```python
from build123d import *

# Parameters (mm, degrees)
ESQUISSE1_W               = 60.5
ESQUISSE1_H               = 64
BOSS_EXTRU_1_DEPTH        = 30
ESQUISSE2_R               = 4.5
ENL_V_MAT_EXTRU_1_DEPTH   = 32
ENL_V_MAT_EXTRU_2_REACH   = 55.283
ESQUISSE4_W               = 51.1
ESQUISSE4_H               = 83.557669167
ESQUISSE5_R               = 10.5
ENL_V_MAT_EXTRU_3_DEPTH   = 2
ESQUISSE6_R               = 10
ENL_V_MAT_EXTRU_4_DEPTH   = 4.7
ESQUISSE7_W               = 47
ESQUISSE7_H               = 57
BOSS_EXTRU_2_DEPTH        = 30
ENL_V_MAT_EXTRU_5_DEPTH   = 30
ENL_V_MAT_EXTRU_6_DEPTH   = 8.25
ESQUISSE11_W              = 5
ESQUISSE11_H              = 40.5
BOSS_EXTRU_3_DEPTH        = 5
ESQUISSE12_R              = 0.5
ENL_V_MAT_EXTRU_7_DEPTH   = 15
TROU_TARAUD_M2X0_42_D     = 1.6
TROU_TARAUD_M2X0_42_DEPTH = 17
TROU_TARAUD_M2X0_42_TIP   = 0.480688495
ENL_V_MAT_EXTRU_8_REACH   = 113.72
ESQUISSE22_W              = 82.97203866
ESQUISSE22_H              = 67.875780224
ENL_V_MAT_EXTRU_10_DEPTH  = 30
ESQUISSE23_W              = 55
ESQUISSE23_H              = 5
ESQUISSE23_H_2            = 4.9
BOSS_EXTRU_4_DEPTH        = 30
ENL_V_START               = -62
ESQUISSE24_R              = 10
ENL_V_MAT_EXTRU_11_DEPTH  = 62
ENL_V_MAT_EXTRU_12_REACH  = 111.597
ESQUISSE26_R              = 10.5
ESQUISSE26_R_2            = 4.5
BOSS_EXTRU_5_DEPTH        = 5
ESQUISSE27_R              = 10.5
ENL_V_MAT_EXTRU_13_DEPTH  = 2.5
ESQUISSE28_W              = 21.53784572
ESQUISSE28_H              = 33.22443827
ENL_V_MAT_EXTRU_14_DEPTH  = 5
ESQUISSE29_W              = 5
ESQUISSE29_H              = 52.1
ENL_V_MAT_EXTRU_15_DEPTH  = 30
BOSS_EXTRU_6_DEPTH        = 62
ENL_V_START_2             = -20.388398
ESQUISSE32_W              = 38.789198293
ESQUISSE32_H              = 52.1
ENL_V_MAT_EXTRU_16_DEPTH  = 20.388398


with BuildPart() as part:
    # Esquisse1 → Boss.-Extru.1 (new body)
    with BuildSketch(Plane.XY):
        Rectangle(ESQUISSE1_W, ESQUISSE1_H)
    extrude(amount=BOSS_EXTRU_1_DEPTH)

    # Esquisse2 → Enlèv. mat.-Extru.1 (cut)
    with BuildSketch(Plane(origin=(30.25, 0, 0), x_dir=(0, 0, -1), z_dir=(1, 0, 0))):
        with Locations(Location((-15, -17, 0), (0, 0, 90))):
            Circle(ESQUISSE2_R)
    extrude(amount=-ENL_V_MAT_EXTRU_1_DEPTH, mode=Mode.SUBTRACT)

    # Enlèv. mat.-Extru.2: up to this face of the body (flat: up to its plane)
    enl_v_mat_extru_2_end = Plane(part.part.faces().sort_by_distance((0, 0, 0))[0])
    # Esquisse4 → Enlèv. mat.-Extru.2 (cut, up to the picked face)
    with BuildSketch(Plane.XY.offset(30), mode=Mode.PRIVATE) as enl_v_mat_extru_2_sk1:
        with Locations((0, -14.778834584)):
            Rectangle(ESQUISSE4_W, ESQUISSE4_H)
    enl_v_mat_extru_2_tool1 = split(extrude(enl_v_mat_extru_2_sk1.sketch, amount=-ENL_V_MAT_EXTRU_2_REACH, mode=Mode.PRIVATE), bisect_by=enl_v_mat_extru_2_end, keep=Keep.BOTH, mode=Mode.PRIVATE)
    add(enl_v_mat_extru_2_tool1.solids().sort_by(Axis((0, -14.778835, 30), (0, 0, -1)))[0], mode=Mode.SUBTRACT)

    # Esquisse5 → Enlèv. mat.-Extru.3 (cut)
    with BuildSketch(Plane(origin=(30.25, 0, 0), x_dir=(0, 0, -1), z_dir=(1, 0, 0))):
        with Locations(Location((-15, -17, 0), (0, 0, 90))):
            Circle(ESQUISSE5_R)
    extrude(amount=-ENL_V_MAT_EXTRU_3_DEPTH, mode=Mode.SUBTRACT)

    # Esquisse6 → Enlèv. mat.-Extru.4 (cut)
    with BuildSketch(Plane(origin=(-25.55, 0, 0), x_dir=(0, 0, -1), z_dir=(1, 0, 0))):
        with Locations((-15, -17)):
            Circle(ESQUISSE6_R)
    extrude(amount=-ENL_V_MAT_EXTRU_4_DEPTH, mode=Mode.SUBTRACT)

    # Esquisse7 → Boss.-Extru.2 (add)
    with BuildSketch(Plane.XY.offset(30)):
        with Locations((-6.75, 60.5)):
            Rectangle(ESQUISSE7_W, ESQUISSE7_H)
    extrude(amount=-BOSS_EXTRU_2_DEPTH)

    # Esquisse8 → Enlèv. mat.-Extru.5 (cut)
    with BuildSketch(Plane.XY.offset(30)):
        Polygon((-15.25, 80.75), (11.75, 80.75), (11.75, 101.149817475), (21.75, 101.149817475), (21.75, 32), (11.75, 32), (11.75, 40.25), (-15.25, 40.25), align=None)
    extrude(amount=-ENL_V_MAT_EXTRU_5_DEPTH, mode=Mode.SUBTRACT)

    # Esquisse10 → Enlèv. mat.-Extru.6 (cut)
    with BuildSketch(Plane.XZ.offset(-80.75)):
        Polygon((-5.25, 11), (-5.25, 12), (34.75, 12), (34.75, 18), (-5.25, 18), (-5.25, 19), (-15.25, 19), (-15.25, 11), align=None)
    extrude(amount=-ENL_V_MAT_EXTRU_6_DEPTH, mode=Mode.SUBTRACT)

    # Esquisse11 → Boss.-Extru.3 (add)
    with BuildSketch(Plane(origin=(-15.25, 0, 0), x_dir=(0, 0, -1), z_dir=(1, 0, 0))):
        with Locations((-27.5, 60.5)):
            Rectangle(ESQUISSE11_W, ESQUISSE11_H)
        with Locations((-2.5, 60.5)):
            Rectangle(ESQUISSE11_W, ESQUISSE11_H)
    extrude(amount=BOSS_EXTRU_3_DEPTH)

    # Esquisse12 → Enlèv. mat.-Extru.7 (cut)
    with BuildSketch(Plane(origin=(11.75, 0, 0), x_dir=(0, 0, -1), z_dir=(1, 0, 0))):
        with Locations((-19.925, 85.21)):
            Circle(ESQUISSE12_R)
        with Locations(Location((-10.075, 85.21, 0), (0, 0, 180))):
            Circle(ESQUISSE12_R)
        with Locations((-10.075, 35.79)):
            Circle(ESQUISSE12_R)
        with Locations(Location((-19.925, 35.79, 0), (0, 0, 180))):
            Circle(ESQUISSE12_R)
    extrude(amount=-ENL_V_MAT_EXTRU_7_DEPTH, mode=Mode.SUBTRACT)

    # Trou taraudé M2x0.42
    with Locations(Plane(origin=(11.75, 85.21, 19.925), x_dir=(0, 0, 1), z_dir=(1, 0, 0))):
        with Locations((0, 0), (-9.85, 0), (-9.85, 49.42), (0, 49.42)):
            Hole(TROU_TARAUD_M2X0_42_D / 2, depth=TROU_TARAUD_M2X0_42_DEPTH)
            with Locations((0, 0, -(TROU_TARAUD_M2X0_42_DEPTH + TROU_TARAUD_M2X0_42_TIP / 2))):  # 118° drill point
                Cone(0, TROU_TARAUD_M2X0_42_D / 2, TROU_TARAUD_M2X0_42_TIP, mode=Mode.SUBTRACT)

    # Enlèv. mat.-Extru.8: up to this face of the body (flat: up to its plane)
    enl_v_mat_extru_8_end = Plane(part.part.faces().sort_by_distance((30.25, 3.741727612, 15))[0])
    # Esquisse15 → Enlèv. mat.-Extru.8 (cut, up to the picked face)
    with BuildSketch(Plane.ZY.offset(30.25), mode=Mode.PRIVATE) as enl_v_mat_extru_8_sk1:
        with BuildLine():
            Line((40, -17), (30, -17))
            ThreePointArc((30, -17), (15, -32), (0, -17))
            Line((0, -17), (-10, -17))
            ThreePointArc((-10, -17), (15, -42), (40, -17))
        make_face()
    enl_v_mat_extru_8_tool1 = split(extrude(enl_v_mat_extru_8_sk1.sketch, amount=-ENL_V_MAT_EXTRU_8_REACH, mode=Mode.PRIVATE), bisect_by=enl_v_mat_extru_8_end, keep=Keep.BOTH, mode=Mode.PRIVATE)
    add(enl_v_mat_extru_8_tool1.solids().sort_by(Axis((-30.25, -17.559017, -5), (1, 0, 0)))[0], mode=Mode.SUBTRACT)

    # Esquisse22 → Enlèv. mat.-Extru.10 (cut)
    with BuildSketch(Plane.XY.offset(30)):
        with Locations((-1.917421061, -6.937890112)):
            Rectangle(ESQUISSE22_W, ESQUISSE22_H)
    extrude(amount=-ENL_V_MAT_EXTRU_10_DEPTH, mode=Mode.SUBTRACT)

    # Esquisse23 → Boss.-Extru.4 (add)
    with BuildSketch(Plane(origin=(0, 0, 0), x_dir=(-1, 0, 0), z_dir=(0, 0, -1))):
        with Locations((57.75, 29.5)):
            Rectangle(ESQUISSE23_W, ESQUISSE23_H)
        with Locations((57.75, 86.55)):
            Rectangle(ESQUISSE23_W, ESQUISSE23_H_2)
    extrude(amount=-BOSS_EXTRU_4_DEPTH)

    # Esquisse24 → Enlèv. mat.-Extru.11 (cut)
    with BuildSketch(Plane.XZ.offset(-27).offset(ENL_V_START)):
        with Locations((-74.25, 15)):
            Circle(ESQUISSE24_R)
    extrude(amount=ENL_V_MAT_EXTRU_11_DEPTH, mode=Mode.SUBTRACT)

    # Enlèv. mat.-Extru.12: up to this face of the body (flat: up to its plane)
    enl_v_mat_extru_12_end = Plane(part.part.faces().sort_by_distance((-34.437928466, 89, 15))[0])
    # Esquisse25 → Enlèv. mat.-Extru.12 (cut, up to the picked face)
    with BuildSketch(Plane.XZ.offset(-27), mode=Mode.PRIVATE) as enl_v_mat_extru_12_sk1:
        with BuildLine():
            Line((-74.25, 44.134833893), (-74.25, 30))
            ThreePointArc((-74.25, 30), (-89.25, 15), (-74.25, 0))
            Line((-74.25, 0), (-74.25, -14.134833893))
            ThreePointArc((-74.25, -14.134833893), (-103.384833893, 15), (-74.25, 44.134833893))
        make_face()
    enl_v_mat_extru_12_tool1 = split(extrude(enl_v_mat_extru_12_sk1.sketch, amount=-ENL_V_MAT_EXTRU_12_REACH, mode=Mode.PRIVATE), bisect_by=enl_v_mat_extru_12_end, keep=Keep.BOTH, mode=Mode.PRIVATE)
    add(enl_v_mat_extru_12_tool1.solids().sort_by(Axis((-74.901475, 27, 37.067417), (0, 1, 0)))[0], mode=Mode.SUBTRACT)

    # Esquisse26 → Boss.-Extru.5 (add)
    with BuildSketch(Plane.XZ.offset(-27)):
        with Locations((-74.25, 15)):
            Circle(ESQUISSE26_R)
        with Locations((-74.25, 15)):
            Circle(ESQUISSE26_R_2, mode=Mode.SUBTRACT)
    extrude(amount=-BOSS_EXTRU_5_DEPTH)

    # Esquisse27 → Enlèv. mat.-Extru.13 (cut)
    with BuildSketch(Plane.XZ.offset(-27)):
        with Locations((-74.25, 15)):
            Circle(ESQUISSE27_R)
    extrude(amount=-ENL_V_MAT_EXTRU_13_DEPTH, mode=Mode.SUBTRACT)

    # Esquisse28 → Enlèv. mat.-Extru.14 (cut)
    with BuildSketch(Plane(origin=(0, 32, 0), x_dir=(1, 0, 0), z_dir=(0, 1, 0))):
        with Locations((22.51892286, -16.612219135)):
            Rectangle(ESQUISSE28_W, ESQUISSE28_H)
    extrude(amount=-ENL_V_MAT_EXTRU_14_DEPTH, mode=Mode.SUBTRACT)

    # Esquisse29 → Enlèv. mat.-Extru.15 (cut)
    with BuildSketch(Plane(origin=(0, 0, 0), x_dir=(-1, 0, 0), z_dir=(0, 0, -1))):
        with Locations((27.75, 58.05)):
            Rectangle(ESQUISSE29_W, ESQUISSE29_H)
    extrude(amount=-ENL_V_MAT_EXTRU_15_DEPTH, mode=Mode.SUBTRACT)

    # Esquisse31 → Boss.-Extru.6 (add)
    with BuildSketch(Plane.XZ.offset(-27)):
        with BuildLine():
            ThreePointArc((-74.826036871, 4.515812787), (-83.84709586, 10.740217019), (-82.411654216, 21.605861069))
            Line((-82.411654216, 21.605861069), (-85.25, 25.198039027))
            Line((-85.25, 25.198039027), (-85.25, 4.801960973))
            Line((-85.25, 4.801960973), (-74.826036871, 4.515812787))
        make_face()
        with BuildLine():
            ThreePointArc((-85.25, 25.198039027), (-89.25, 15), (-85.25, 4.801960973))
            Line((-85.25, 4.801960973), (-85.25, 25.198039027))
        make_face()
    extrude(amount=-BOSS_EXTRU_6_DEPTH)

    # Esquisse32 → Enlèv. mat.-Extru.16 (cut)
    with BuildSketch(Plane(origin=(0.067526976, 0, 2.459909751), x_dir=(-0.9996234341769173, 0, 0.027440660421105302), z_dir=(-0.027440660421105302, 0, -0.9996234341769173)).offset(ENL_V_START_2)):
        with Locations((94.316375975, 58.05)):
            Rectangle(ESQUISSE32_W, ESQUISSE32_H)
    extrude(amount=ENL_V_MAT_EXTRU_16_DEPTH, mode=Mode.SUBTRACT)


solid = part.part
```
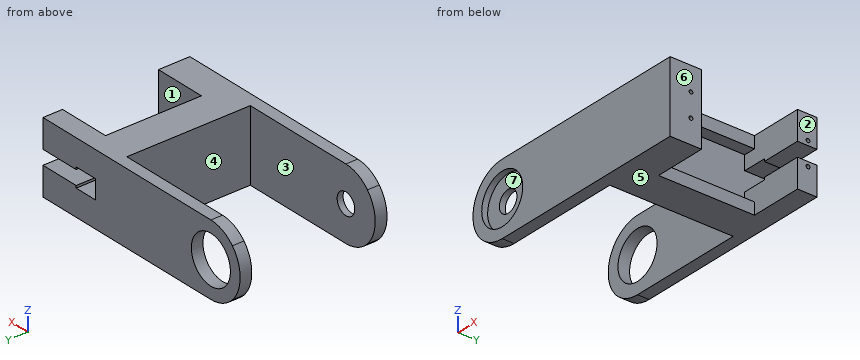
For this review, take the finished solid that the model builds, in its own axes (mm). Face numbers are marked on the shaded views. A direction names the side the tool comes from. Round coordinates to 2 decimals unless told otherwise and drop trailing zeros. Write each loop counter-clockwise with the first axis right and the second up, starting at its lowest first coordinate (ties: lowest second). Pieces come first, ordered by that corner, then holes. Notation, with made-up numbers: (-9.5, 41) -> (24.5, 41) arc R28 cw to (24.5, 75) -> close; hole circle Ø9 at (-17.75, -33.75). An arc over 180 degrees is marked (long way). One line per question, with ' | ' between items. Start each with the question number.
1) Add section D-D (y = 71). Write out the cut boundary in (x, z).
2) Add section C-C (z = 8). Write out the cut boundary in (x, y).
3) Add section A-A (x = 4.5). Write out the cut boundary in (y, z) (3 decimals), and give its area (3 significant figures).
4) Mouldability with a two-part tool opening along X and no side actions: class the marked faces 4, 5, 6 and 7 as +X half, -X half, draft (parallel to the pull), parting line (faces both ways), or undercut.
5) Wall thickness on line 1 along Z through (x, y) = (2, 85.21) (3 decimals); line 2 along Y through (x, z) = (0, 27.25); line 3 along Y through (x, z) = (-62.5, 21.25): over which ranges is each line inside the solid? List them lowest first.
6) For pin 1 Ø1.3 at (y, z) = (35.79, 10.075) entering from -X; pin 2 Ø16 at (x, z) = (-74.25, 15) entering from -Y; pin 3 Ø5.5 at (y, z) = (70.5, 1.5) entering from +X; pin 4 Ø10 at (x, y) = (-5, 60) entering from -Z, all flat-tipped, find the tip position at first contact; note any pin that passes through.
7) Machinability: for the marked faces 1, 2 and 3, which of the approach directions +Z, -Z, +X, -X, +Y, -Y give a long, thin tool a straight path to every point of the face, cutting with its end or side? Answer none if there is none.
8) Add section B-B (x = -58). Write out the cut boundary in (y, z).
Reported:
1) outline: (-25.25, 0) -> (-10.25, 0) -> (-10.25, 5) -> (-15.25, 5) -> (-15.25, 25) -> (-10.25, 25) -> (-10.25, 30) -> (-25.25, 30) -> close
2) outline: (-87.52, 27) -> (-82.08, 27) -> (-82.08, 29.5) -> (-66.42, 29.5) -> (-66.42, 27) -> (11.75, 27) -> (11.75, 40.25) -> (-15.25, 40.25) -> (-15.25, 80.75) -> (11.75, 80.75) -> (11.75, 89) -> (-67.11, 89) -> (-67.11, 84.1) -> (-25.25, 84.1) -> (-25.25, 32) -> (-87.52, 32) -> close; (-87.52, 84.1) -> (-81.39, 84.1) -> (-81.39, 89) -> (-87.52, 89) -> close
3) outline: (27, 0) -> (40.25, 0) -> (40.25, 30) -> (27, 30) -> close; (80.75, 0) -> (89, 0) -> (89, 12) -> (80.75, 12) -> close; (80.75, 18) -> (89, 18) -> (89, 30) -> (80.75, 30) -> close; hole circle Ø1.6 at (35.79, 10.075); hole circle Ø1.6 at (35.79, 19.925); hole circle Ø1.6 at (85.21, 10.075); hole circle Ø1.6 at (85.21, 19.925) | area: 587 mm²
4) face 4: -X half | face 5: draft | face 6: +X half | face 7: undercut
5) line 1: z = 0 to 9.275, 10.875 to 12, 18 to 19.125, 20.725 to 30 | line 2: y = 27 to 40.25, 80.75 to 89 | line 3: y = 27 to 32, 84.1 to 89
6) pin 1: stops at x = -25.25 | pin 2: stops at y = 29.5 | pin 3: stops at x = -10.25 | pin 4: passes through
7) face 1: +X | face 2: +Z, -Z, +X, +Y, -Y | face 3: +Z, -Z, -X
8) outline: (27, 0) -> (32, 0) -> (32, 30) -> (27, 30) -> close; (84.1, 0) -> (89, 0) -> (89, 30) -> (84.1, 30) -> close
